For this review, take the finished solid that the model builds, in its own axes (mm). Round coordinates to 2 decimals unless told otherwise and drop trailing zeros. Write each loop counter-clockwise with the first axis right and the second up, starting at its lowest first coordinate (ties: lowest second). Pieces come first, ordered by that corner, then holes. Notation, with made-up numbers: M 37.5,12 L 61.5,12 A11 cw 61.5,27 Z; hole C 78.5,-19 d4. An arc over 180 degrees is marked long. One line per question, with ' | ' between items.
```python
from build123d import *

# Parameters (mm, degrees)
SKETCH1_R           = 0.8
BOSS_EXTRUDE1_DEPTH = 2


with BuildPart() as part:
    # Sketch1 → Boss-Extrude1 (new body)
    with BuildSketch(Plane(origin=(0, 0, 0), x_dir=(1, 0, 0), z_dir=(0, 1, 0))):
        with BuildLine():
            Line((1, 0), (5, 0))
            ThreePointArc((5, 0), (5.707106781, -0.292893219), (6, -1))
            Line((6, -1), (6, -5))
            Line((6, -5), (7, -5))
            Line((7, -5), (7, -25))
            Line((7, -25), (15, -25))
            Line((15, -25), (15, 2.965311532))
            Line((15, 2.965311532), (4.948577491, 14.065616497))
            ThreePointArc((4.948577491, 14.065616497), (1.819757882, 14.809804225), (0, 12.158048434))
            Line((0, 12.158048434), (0, 1))
            ThreePointArc((0, 1), (0.292893219, 0.292893219), (1, 0))
        make_face()
        with Locations(Location((2.841951566, 7.561679983, 0), (0, 0, 270))):
            Circle(SKETCH1_R, mode=Mode.SUBTRACT)
        with Locations(Location((2.841951566, 2.965311532, 0), (0, 0, 270))):
            Circle(SKETCH1_R, mode=Mode.SUBTRACT)
        with Locations(Location((2.841951566, 12.158048434, 0), (0, 0, 270))):
            Circle(SKETCH1_R, mode=Mode.SUBTRACT)
    extrude(amount=BOSS_EXTRUDE1_DEPTH)


solid = part.part
```
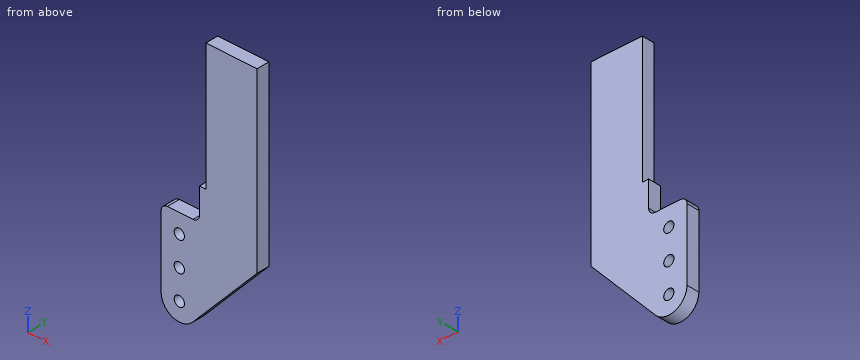
Item 1: Insertion check: pin 1 Ø0.6 at (y, z) = (1, 12.5) entering from -X; pin 2 Ø0.6 at (x, y) = (3.5, 1) entering from +Z. Each pin has a flat end and moves straight along its axis. Give the tip position at first contact, or say it passes through.
Results:
pin 1: x = 7 | pin 2: z = 0
Item 2: To check wall thickness, follow line 1 along X through (y, z) = (1.55, 5.5); line 2 along Z through (x, y) = (2.5, 0.4); line 3 along X through (y, z) = (1.7, -8). State the ranges of each line that lie inside material, in increasing order. Write a range as from..to.
Results:
line 1: 7..15 | line 2: -14.98..-12.88, -11.43..-8.28, -6.84..-3.69, -2.24..0 | line 3: 0..2.17, 3.51..10.44
Item 3: Take a section at A-A (y = 0.7). Write out the cut boundary in (x, z), then the cut area to 3 significant figures.
Results:
outline: M 0,-12.16 A2.84 ccw 4.95,-14.07 L 15,-2.97 L 15,25 L 7,25 L 7,5 L 6,5 L 6,1 A1 cw 5,0 L 1,0 A1 ccw 0,-1 Z; hole C 2.84,-12.16 d1.6; hole C 2.84,-7.56 d1.6; hole C 2.84,-2.97 d1.6 | area: 356 mm2
Item 4: Take a section at B-B (z = 13.5). Write out the cut boundary in (x, y).
Results:
outline: M 7,0 L 15,0 L 15,2 L 7,2 Z
Item 5: Take a section at C-C (x = 13.5). Write out the cut boundary in (y, z).
Results:
outline: M 0,-4.62 L 2,-4.62 L 2,25 L 0,25 Z
